```python
from build123d import *

# Parameters (mm, degrees)
EXTRUDE_1_DEPTH     = 20
CUT_EXTRUDE_1_DEPTH = 20
SKETCH_3_R          = 5
CUT_EXTRUDE_2_DEPTH = 3
CUT_EXTRUDE_3_DEPTH = 6
SKETCH_5_R          = 5
CUT_EXTRUDE_4_DEPTH = 3
SKETCH_6_W          = 90
SKETCH_6_H          = 20
EXTRUDE_2_DEPTH     = 6
SKETCH_7_R          = 5
CUT_EXTRUDE_5_DEPTH = 3
SKETCH_8_R          = 2.6
CUT_EXTRUDE_6_DEPTH = 3
SKETCH_11_W         = 118.79393924
SKETCH_11_H         = 4
EXTRUDE_4_DEPTH     = 4
SKETCH_12_W         = 110
SKETCH_12_H         = 4
EXTRUDE_5_DEPTH     = 4
SKETCH_13_W         = 20
SKETCH_13_H         = 4
EXTRUDE_6_DEPTH     = 4
FILLET_2_R          = 12
FILLET_3_R          = 50
SKETCH_14_W         = 4
SKETCH_14_H         = 12
EXTRUDE_7_DEPTH     = 4


with BuildPart() as part:
    # 草图1 → 凸台-拉伸1 (new body)
    with BuildSketch(Plane(origin=(0, 0, 0), x_dir=(1, 0, 0), z_dir=(0, 1, 0))):
        Polygon((0, 0), (110, 0), (110, -6), (90, -6), (6, -90), (6, -110), (0, -110), align=None)
    extrude(amount=EXTRUDE_1_DEPTH)

    # 草图2 → 切除-拉伸1 (cut)
    with BuildSketch(Plane(origin=(6, 0, 0), x_dir=(0, 0, -1), z_dir=(1, 0, 0))):
        with BuildLine():
            ThreePointArc((-97.4, 10), (-99.005023076, 12.402086785), (-101.838477631, 11.838477631))
            Line((-101.838477631, 11.838477631), (-98.161522369, 8.161522369))
            ThreePointArc((-98.161522369, 8.161522369), (-97.597913215, 9.005023076), (-97.4, 10))
        make_face()
        with BuildLine():
            Line((-98.161522369, 8.161522369), (-101.838477631, 11.838477631))
            ThreePointArc((-101.838477631, 11.838477631), (-101.838477631, 8.161522369), (-98.161522369, 8.161522369))
        make_face()
    extrude(amount=-CUT_EXTRUDE_1_DEPTH, mode=Mode.SUBTRACT)

    # 草图3 → 切除-拉伸2 (cut)
    with BuildSketch(Plane(origin=(6, 0, 0), x_dir=(0, 0, -1), z_dir=(1, 0, 0))):
        with Locations((-100, 10)):
            Circle(SKETCH_3_R)
    extrude(amount=-CUT_EXTRUDE_2_DEPTH, mode=Mode.SUBTRACT)

    # 草图4 → 切除-拉伸3 (cut)
    with BuildSketch(Plane.XY.offset(6)):
        with BuildLine():
            ThreePointArc((102.6, 10), (100.994976924, 12.402086785), (98.161522369, 11.838477631))
            Line((98.161522369, 11.838477631), (101.838477631, 8.161522369))
            ThreePointArc((101.838477631, 8.161522369), (102.402086785, 9.005023076), (102.6, 10))
        make_face()
        with BuildLine():
            Line((101.838477631, 8.161522369), (98.161522369, 11.838477631))
            ThreePointArc((98.161522369, 11.838477631), (98.161522369, 8.161522369), (101.838477631, 8.161522369))
        make_face()
    extrude(amount=-CUT_EXTRUDE_3_DEPTH, mode=Mode.SUBTRACT)

    # 草图5 → 切除-拉伸4 (cut)
    with BuildSketch(Plane.XY.offset(6)):
        with Locations((100, 10)):
            Circle(SKETCH_5_R)
    extrude(amount=-CUT_EXTRUDE_4_DEPTH, mode=Mode.SUBTRACT)

    # 草图6 → 凸台-拉伸2 (add)
    with BuildSketch(Plane.ZY):
        with Locations((155, 10)):
            Rectangle(SKETCH_6_W, SKETCH_6_H)
    extrude(amount=-EXTRUDE_2_DEPTH)

    # 草图7 → 切除-拉伸5 (cut)
    with BuildSketch(Plane(origin=(6, 0, 0), x_dir=(0, 0, -1), z_dir=(1, 0, 0))):
        with Locations((-190, 10)):
            Circle(SKETCH_7_R)
    extrude(amount=-CUT_EXTRUDE_5_DEPTH, mode=Mode.SUBTRACT)

    # 草图8 → 切除-拉伸6 (cut)
    with BuildSketch(Plane(origin=(3, 0, 0), x_dir=(0, 0, -1), z_dir=(1, 0, 0))):
        with Locations((-190, 10)):
            Circle(SKETCH_8_R)
    extrude(amount=-CUT_EXTRUDE_6_DEPTH, mode=Mode.SUBTRACT)

    # 草图11 → 凸台-拉伸4 (add)
    with BuildSketch(Plane(origin=(48, 0, 48), x_dir=(0.7071067811865475, 0, -0.7071067811865476), z_dir=(0.7071067811865476, 0, 0.7071067811865475))):
        with Locations((0, 18)):
            Rectangle(SKETCH_11_W, SKETCH_11_H)
        with Locations((0, 2)):
            Rectangle(SKETCH_11_W, SKETCH_11_H)
    extrude(amount=EXTRUDE_4_DEPTH)

    # 草图12 → 凸台-拉伸5 (add)
    with BuildSketch(Plane(origin=(6, 0, 0), x_dir=(0, 0, -1), z_dir=(1, 0, 0))):
        with Locations((-145, 18)):
            Rectangle(SKETCH_12_W, SKETCH_12_H)
        with Locations((-145, 2)):
            Rectangle(SKETCH_12_W, SKETCH_12_H)
    extrude(amount=EXTRUDE_5_DEPTH)

    # 草图13 → 凸台-拉伸6 (add)
    with BuildSketch(Plane.XY.offset(6)):
        with Locations((100, 18)):
            Rectangle(SKETCH_13_W, SKETCH_13_H)
        with Locations((100, 2)):
            Rectangle(SKETCH_13_W, SKETCH_13_H)
    extrude(amount=EXTRUDE_6_DEPTH)

    # 圆角2
    fillet_2_edges = [part.edges().sort_by_distance(p)[0] for p in [
        (90, 10, 6),
        (6, 10, 90),
    ]]
    fillet(fillet_2_edges, radius=FILLET_2_R)

    # 圆角3
    # the kernel refuses this fillet: 50 mm, written as the material it adds along each edge
    with BuildSketch(Plane(origin=(10, 0, 91.656854249), x_dir=(0, 0, 1), z_dir=(0, 1, 0))) as fillet_3_piece_1:
        with BuildLine():
            CenterArc((FILLET_3_R * 0.414213562373, FILLET_3_R), FILLET_3_R, 225, 45)
            Line((-FILLET_3_R * 0.292893218813, FILLET_3_R * 0.292893218813), (-FILLET_3_R * 0.307035354437, FILLET_3_R * 0.27875108319))
            Line((-FILLET_3_R * 0.307035354437, FILLET_3_R * 0.27875108319), (-FILLET_3_R * 0.00828427124746, -FILLET_3_R * 0.02))
            Line((-FILLET_3_R * 0.00828427124746, -FILLET_3_R * 0.02), (FILLET_3_R * 0.414213562373, -FILLET_3_R * 0.02))
            Line((FILLET_3_R * 0.414213562373, -FILLET_3_R * 0.02), (FILLET_3_R * 0.414213562373, 0))
        make_face()
    extrude(amount=4)
    with BuildSketch(Plane(origin=(10, 0, 91.656854249), x_dir=(0, 0, 1), z_dir=(0, 1, 0))) as fillet_3_piece_2_section:
        with BuildLine():
            CenterArc((FILLET_3_R * 0.414213562373, FILLET_3_R), FILLET_3_R, 225, 45)
            Line((-FILLET_3_R * 0.292893218813, FILLET_3_R * 0.292893218813), (-FILLET_3_R * 0.307035354437, FILLET_3_R * 0.27875108319))
            Line((-FILLET_3_R * 0.307035354437, FILLET_3_R * 0.27875108319), (-FILLET_3_R * 0.00828427124746, -FILLET_3_R * 0.02))
            Line((-FILLET_3_R * 0.00828427124746, -FILLET_3_R * 0.02), (FILLET_3_R * 0.414213562373, -FILLET_3_R * 0.02))
            Line((FILLET_3_R * 0.414213562373, -FILLET_3_R * 0.02), (FILLET_3_R * 0.414213562373, 0))
        make_face()
    fillet_3_piece_2 = extrude(amount=55.776695297, mode=Mode.PRIVATE)
    fillet_3_piece_2 = split(fillet_3_piece_2, bisect_by=Plane(origin=(13.090507107, 16, 92.936984208), z_dir=(0, 1, 0)), keep=Keep.TOP, mode=Mode.PRIVATE)
    fillet_3_piece_2 = split(fillet_3_piece_2, bisect_by=Plane(origin=(13.090507107, 20, 92.936984208), z_dir=(0, -1, 0)), keep=Keep.TOP, mode=Mode.PRIVATE)
    add(fillet_3_piece_2)
    with BuildSketch(Plane(origin=(10, 20, 91.656854249), x_dir=(0, 0, 1), z_dir=(0, -1, 0))) as fillet_3_piece_3:
        with BuildLine():
            CenterArc((FILLET_3_R * 0.414213562373, -FILLET_3_R), FILLET_3_R, 90, 45)
            Line((-FILLET_3_R * 0.292893218813, -FILLET_3_R * 0.292893218813), (-FILLET_3_R * 0.307035354437, -FILLET_3_R * 0.27875108319))
            Line((-FILLET_3_R * 0.307035354437, -FILLET_3_R * 0.27875108319), (-FILLET_3_R * 0.00828427124746, FILLET_3_R * 0.02))
            Line((-FILLET_3_R * 0.00828427124746, FILLET_3_R * 0.02), (FILLET_3_R * 0.414213562373, FILLET_3_R * 0.02))
            Line((FILLET_3_R * 0.414213562373, FILLET_3_R * 0.02), (FILLET_3_R * 0.414213562373, 0))
        make_face()
    extrude(amount=4)
    with BuildSketch(Plane(origin=(10, 20, 91.656854249), x_dir=(0, 0, 1), z_dir=(0, -1, 0))) as fillet_3_piece_4_section:
        with BuildLine():
            CenterArc((FILLET_3_R * 0.414213562373, -FILLET_3_R), FILLET_3_R, 90, 45)
            Line((-FILLET_3_R * 0.292893218813, -FILLET_3_R * 0.292893218813), (-FILLET_3_R * 0.307035354437, -FILLET_3_R * 0.27875108319))
            Line((-FILLET_3_R * 0.307035354437, -FILLET_3_R * 0.27875108319), (-FILLET_3_R * 0.00828427124746, FILLET_3_R * 0.02))
            Line((-FILLET_3_R * 0.00828427124746, FILLET_3_R * 0.02), (FILLET_3_R * 0.414213562373, FILLET_3_R * 0.02))
            Line((FILLET_3_R * 0.414213562373, FILLET_3_R * 0.02), (FILLET_3_R * 0.414213562373, 0))
        make_face()
    fillet_3_piece_4 = extrude(amount=55.776695297, mode=Mode.PRIVATE)
    fillet_3_piece_4 = split(fillet_3_piece_4, bisect_by=Plane(origin=(13.090507107, 4, 92.936984208), z_dir=(0, -1, 0)), keep=Keep.TOP, mode=Mode.PRIVATE)
    fillet_3_piece_4 = split(fillet_3_piece_4, bisect_by=Plane(origin=(13.090507107, 0, 92.936984208), z_dir=(0, 1, 0)), keep=Keep.TOP, mode=Mode.PRIVATE)
    add(fillet_3_piece_4)
    with BuildSketch(Plane(origin=(91.656854249, 0, 10), x_dir=(1, 0, 0), z_dir=(0, 1, 0))) as fillet_3_piece_5:
        with BuildLine():
            CenterArc((20.769589097, -49.941089022), FILLET_3_R, 92.781591787, 42.218408213)
            Line((-14.585749963, -14.585749963), (-15.292856744, -13.878643181))
            Line((-15.292856744, -13.878643181), (-0.707106781, 0.707106781))
            Line((-0.707106781, 0.707106781), (0, 1))
            ThreePointArc((0, 1), (9.171572875, 1), (18.294616884, 0.99882178))
            Line((18.294616884, 0.99882178), (18.343145751, 0))
        make_face()
    extrude(amount=4)
    with BuildSketch(Plane(origin=(91.656854249, 0, 10), x_dir=(1, 0, 0), z_dir=(0, 1, 0))) as fillet_3_piece_6_section:
        with BuildLine():
            CenterArc((20.769589097, -49.941089022), FILLET_3_R, 92.781591787, 42.218408213)
            Line((-14.585749963, -14.585749963), (-15.292856744, -13.878643181))
            Line((-15.292856744, -13.878643181), (-0.707106781, 0.707106781))
            Line((-0.707106781, 0.707106781), (0, 1))
            ThreePointArc((0, 1), (9.171572875, 1), (18.294616884, 0.99882178))
            Line((18.294616884, 0.99882178), (18.343145751, 0))
        make_face()
    fillet_3_piece_6 = extrude(amount=55.568413536, mode=Mode.PRIVATE)
    fillet_3_piece_6 = split(fillet_3_piece_6, bisect_by=Plane(origin=(92.410386276, 16, 13.180383565), z_dir=(0, 1, 0)), keep=Keep.TOP, mode=Mode.PRIVATE)
    fillet_3_piece_6 = split(fillet_3_piece_6, bisect_by=Plane(origin=(92.410386276, 20, 13.180383565), z_dir=(0, -1, 0)), keep=Keep.TOP, mode=Mode.PRIVATE)
    add(fillet_3_piece_6)
    with BuildSketch(Plane(origin=(91.656854249, 20, 10), x_dir=(1, 0, 0), z_dir=(0, -1, 0))) as fillet_3_piece_7:
        with BuildLine():
            CenterArc((20.769589097, 49.941089022), FILLET_3_R, 225, 42.218408213)
            Line((-14.585749963, 14.585749963), (-15.292856744, 13.878643181))
            Line((-15.292856744, 13.878643181), (-0.707106781, -0.707106781))
            Line((-0.707106781, -0.707106781), (0, -1))
            ThreePointArc((0, -1), (9.171572875, -1), (18.294616884, -0.99882178))
            Line((18.294616884, -0.99882178), (18.343145751, 0))
        make_face()
    extrude(amount=4)
    with BuildSketch(Plane(origin=(91.656854249, 20, 10), x_dir=(1, 0, 0), z_dir=(0, -1, 0))) as fillet_3_piece_8_section:
        with BuildLine():
            CenterArc((20.769589097, 49.941089022), FILLET_3_R, 225, 42.218408213)
            Line((-14.585749963, 14.585749963), (-15.292856744, 13.878643181))
            Line((-15.292856744, 13.878643181), (-0.707106781, -0.707106781))
            Line((-0.707106781, -0.707106781), (0, -1))
            ThreePointArc((0, -1), (9.171572875, -1), (18.294616884, -0.99882178))
            Line((18.294616884, -0.99882178), (18.343145751, 0))
        make_face()
    fillet_3_piece_8 = extrude(amount=55.568413536, mode=Mode.PRIVATE)
    fillet_3_piece_8 = split(fillet_3_piece_8, bisect_by=Plane(origin=(92.410386276, 4, 13.180383565), z_dir=(0, -1, 0)), keep=Keep.TOP, mode=Mode.PRIVATE)
    fillet_3_piece_8 = split(fillet_3_piece_8, bisect_by=Plane(origin=(92.410386276, 0, 13.180383565), z_dir=(0, 1, 0)), keep=Keep.TOP, mode=Mode.PRIVATE)
    add(fillet_3_piece_8)

    # 草图14 → 凸台-拉伸7 (add)
    with BuildSketch(Plane(origin=(6, 0, 0), x_dir=(0, 0, -1), z_dir=(1, 0, 0))):
        with Locations((-198, 10)):
            Rectangle(SKETCH_14_W, SKETCH_14_H)
    extrude(amount=EXTRUDE_7_DEPTH)


solid = part.part
```
Verification items for the finished model (mm, model axes). A direction names the side the tool comes from. Round coordinates to 2 decimals unless told otherwise and drop trailing zeros. Write each loop counter-clockwise with the first axis right and the second up, starting at its lowest first coordinate (ties: lowest second). Pieces come first, ordered by that corner, then holes. Notation, with made-up numbers: (38.5, 65) -> (71.5, 65) arc R16 cw to (71.5, 72) -> close; hole circle Ø2 at (-17, -26). An arc over 180 degrees is marked (long way). Write each question's results on one line, items separated by ' | '.
Q1. Draft check along Z on faces 6 (the face through (27, 16, 72)), 7 (the face through (102, 8, 3)), 8 (the face through (10, 17, 157)), 9 (the face through (54, 10, 0)). Enter one of: released by +Z, released by -Z, zero draft, split by the parting line, or undercut.
Derived:
face 6: undercut | face 7: released by +Z | face 8: zero draft | face 9: released by -Z
Q2. Sectioned sample at A-A, the plane z = 119. Record the boundary of the cut face in (x, y).
Derived:
outline: (0, 0) -> (10, 0) -> (10, 4) -> (6, 4) -> (6, 16) -> (10, 16) -> (10, 20) -> (0, 20) -> close
Q3. Sectioned sample at C-C, the plane x = 14.5. Record the boundary of the cut face in (y, z), and give its area (3 significant figures).
Derived:
outline: (0, 0) -> (20, 0) -> (20, 91.64) -> (16, 91.64) -> (16, 81.5) -> (4, 81.5) -> (4, 91.64) -> (0, 91.64) -> close | area: 1,710 mm²
Q4. Sectioned sample at B-B, the plane x = 100. Record the boundary of the cut face in (y, z).
Derived:
outline: (0, 0) -> (7.4, 0) -> (7.4, 3) -> (5, 3) -> (5, 6) -> (4, 6) -> (4, 11.51) -> (0, 11.51) -> close; (12.6, 0) -> (20, 0) -> (20, 11.51) -> (16, 11.51) -> (16, 6) -> (15, 6) -> (15, 3) -> (12.6, 3) -> close
Q5. Thickness scan on probe 1 along Y at (x, z) = (1, 190); probe 2 along Y at (x, z) = (4.85, 100); probe 3 along X at (y, z) = (16.25, 129). Record the ranges inside material, lowest first.
Derived:
probe 1: y = 0 to 7.4, 12.6 to 20 | probe 2: y = 0 to 5, 15 to 20 | probe 3: x = 0 to 10
Q6. Go/stop test with flat-tipped pins: pin 1 Ø5 at (x, y) = (101, 12.5) entering from +Z; pin 2 Ø3 at (y, z) = (7.5, 115) entering from +X; pin 3 Ø3 at (y, z) = (12, 98.5) entering from +X; pin 4 Ø4.5 at (y, z) = (10, 190) entering from -X. Record where each tip stops, or that it passes through.
Derived:
pin 1: stops at z = 6 | pin 2: stops at x = 6 | pin 3: stops at x = 3 | pin 4: passes through
Q7. Access from +Z, -Z, +X, -X, +Y, -Y to the whole of each face (thin tool, end or side, straight path). Record for faces 1 (the face through (1.5, 9, 187.6)), 2 (the face through (50.491, 2.028, 51.166)), 3 (the face through (104.619, 8.085, 4.521)), 4 (the face through (3, 8, 188)), 5 (the face through (106, 10, 6)).
Derived:
face 1: +X, -X | face 2: +Z, +X, +Y, -Y | face 3: +Z | face 4: +X | face 5: +Z, +X
